Here's how the part is built. I have some questions about the finished solid (model axes, mm). Face numbers are marked on the shaded views. Round coordinates to 2 decimals unless told otherwise and drop trailing zeros. Order: outer loops, then holes, each group sorted by start corner. A loop starts at its lowest first (then second) coordinate and runs counter-clockwise, first axis right, second up. Notation, with made-up numbers: (-19.5, -36) -> (38.5, -36) arc R11 cw to (38.5, -16) -> close; hole circle Ø7 at (-10, -30.75). An arc over 180 degrees is marked (long way). Use a Markdown table: item, result. Add a question column.
(1) I want a section at C-C, the plane z = 38. Please give me the cut outline in (x, y).
(2) Thinking about a two-plate mould opening in Y: for the marked faces 1, 2 and 3, which applies, pulls with the +Y half, pulls with the -Y half, needs draft (parallel to the pull), parting line crosses it, or undercut?
(3) If I drill on probe 1 along X at (y, z) = (-21.5, -14); probe 2 along Z at (x, y) = (22.75, 35); probe 3 along Z at (x, y) = (28, 6.5), over which ranges is the centre line in solid material (lowest first)?
(4) I want a section at A-A, the plane y = 0. Please give me the cut outline in (x, z), then the cut area to 3 significant figures.
(5) I want a section at B-B, the plane z = 0. Give the number of separate pieces and of enclosed holes in the cut face, then the cut area to 3 significant figures.
(6) I'm going to push flat-ended pins straight in: P1, Ø10.5, axis at y = 29.12, z = 50.44, coming from the +X side; P2, Ø2.5, axis at y = -29.5, z = 48.5, coming from the +X side; P3, Ø6.5, axis at y = 58.24, z = 0, coming from the -X side; P4, Ø4.5, axis at y = -58.24, z = 0, coming from the -X side. Where does each tip first touch, or does it pass through?
(7) I want a section at D-D, the plane y = 45.5. Please give me the cut outline in (x, z), then the cut area to 3 significant figures.
from build123d import *

# Parameters (mm, degrees)
CUT_EXTRUDE1_START = 24.0348
SKETCH7_R          = 3.96875
CUT_EXTRUDE1_DEPTH = 1.905
SKETCH8_R          = 2.38125
CUT_EXTRUDE2_DEPTH = 35.809800078


with BuildPart() as part:
    # Sketch3 → Revolve1 (revolve)
    with BuildSketch(Plane.XY):
        Polygon((34.809800078, 25.000000038), (34.809800078, 22.999999974), (31.309800093, 19.499999989), (29.909799972, 19.499999989), (29.909799972, 21.000000037), (22.939799942, 21.000000037), (22.939799942, 51.308), (21.469400038, 51.308), (21.469400038, 63.5), (25.939800038, 63.5), (25.939800038, 25.000000038), (27.839800048, 25.000000038), align=None)
    revolve(axis=Axis((0, 0, 0), (1, 0, 0)))

    # Sketch7 → Cut-Extrude1 (cut)
    with BuildSketch(Plane(origin=(0, 0, 0), x_dir=(0, 0, -1), z_dir=(1, 0, 0)).offset(CUT_EXTRUDE1_START)):
        with Locations((50.436020463, -29.119249991)):
            Circle(SKETCH7_R)
        with Locations((0, -58.238499982)):
            Circle(SKETCH7_R)
        with Locations((-50.436020463, -29.119249991)):
            Circle(SKETCH7_R)
        with Locations((-50.436020463, 29.119249991)):
            Circle(SKETCH7_R)
        with Locations((50.436020463, 29.119249991)):
            Circle(SKETCH7_R)
        with Locations((0, 58.238499982)):
            Circle(SKETCH7_R)
    extrude(amount=CUT_EXTRUDE1_DEPTH, mode=Mode.SUBTRACT)

    # Sketch8 → Cut-Extrude2 (cut, through all)
    with BuildSketch(Plane(origin=(0, 0, 0), x_dir=(0, 0, -1), z_dir=(1, 0, 0))):
        with Locations((50.436020463, 29.119249991)):
            Circle(SKETCH8_R)
        with Locations((50.436020463, -29.119249991)):
            Circle(SKETCH8_R)
        with Locations((0, -58.238499982)):
            Circle(SKETCH8_R)
        with Locations((-50.436020463, -29.119249991)):
            Circle(SKETCH8_R)
        with Locations((-50.436020463, 29.119249991)):
            Circle(SKETCH8_R)
        with Locations((0, 58.238499982)):
            Circle(SKETCH8_R)
    extrude(amount=CUT_EXTRUDE2_DEPTH, mode=Mode.SUBTRACT)


solid = part.part
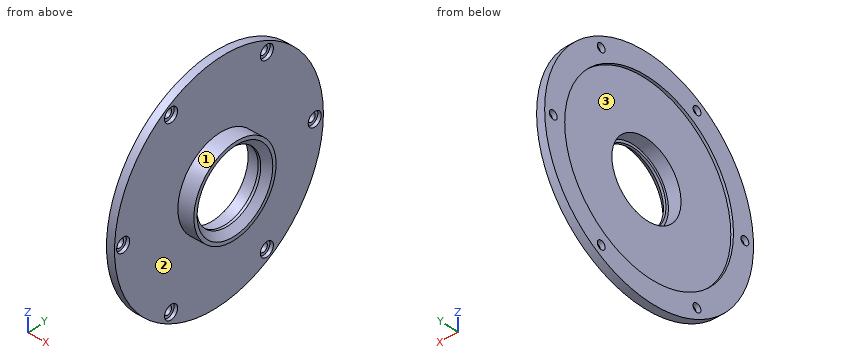
Taken from the geometry:
| question | item | result |
|---|---|---|
| 1 | outline | (21.47, -50.87) -> (25.94, -50.87) -> (25.94, 50.87) -> (21.47, 50.87) -> (21.47, 34.47) -> (22.94, 34.47) -> (22.94, -34.47) -> (21.47, -34.47) -> close |
| 2 | face 1 | parting line crosses it |
| 2 | face 2 | needs draft |
| 2 | face 3 | undercut |
| 3 | probe 1 | x = 22.94 to 25.94 |
| 3 | probe 2 | z = -52.98 to -37.52, 37.52 to 52.98 |
| 3 | probe 3 | z = -24.14 to -19.97, 19.97 to 24.14 |
| 4 | outline | (21.47, -63.5) -> (25.94, -63.5) -> (25.94, -25) -> (34.81, -25) -> (34.81, -23) -> (31.31, -19.5) -> (29.91, -19.5) -> (29.91, -21) -> (22.94, -21) -> (22.94, -51.31) -> (21.47, -51.31) -> close; (21.47, 51.31) -> (22.94, 51.31) -> (22.94, 21) -> (29.91, 21) -> (29.91, 19.5) -> (31.31, 19.5) -> (34.81, 23) -> (34.81, 25) -> (25.94, 25) -> (25.94, 63.5) -> (21.47, 63.5) -> close |
| 4 | area | 364 mm2 |
| 5 | separate pieces | 4 |
| 5 | enclosed holes | 0 |
| 5 | area | 310 mm2 |
| 6 | P1 | stops at x = 25.94 |
| 6 | P2 | stops at x = 24.03 |
| 6 | P3 | stops at x = 21.47 |
| 6 | P4 | passes through |
| 7 | outline | (21.47, -44.29) -> (25.94, -44.29) -> (25.94, 44.29) -> (21.47, 44.29) -> (21.47, 23.71) -> (22.94, 23.71) -> (22.94, -23.71) -> (21.47, -23.71) -> close |
| 7 | area | 326 mm2 |
